from build123d import *

# Parameters (mm, degrees)
BOSS_EXTRUDE1_DEPTH             = 4
SKETCH2_W                       = 7.077783737
SKETCH2_H                       = 4
CUT_EXTRUDE1_DEPTH              = 2.402922374
BOSS_EXTRUDE2_START             = 4
BOSS_EXTRUDE2_DEPTH             = 4
SKETCH4_W                       = 7.077783737
SKETCH4_H                       = 8
CUT_EXTRUDE2_DEPTH              = 14.891763442
BOSS_EXTRUDE3_DEPTH             = 4
CUT_EXTRUDE3_DEPTH              = 6
SCALE1_SCALE                    = 0.6
SCALE2_SCALE                    = 1.1
CHAMFER2_ANGLE                  = 32.170804
CHAMFER3_ANGLE                  = 32.170804
CHAMFER4_ANGLE                  = 37.089833
SKETCH9_W                       = 9.052660039
SKETCH9_H                       = 40.26
BOSS_EXTRUDE4_DEPTH             = 10
BOSS_EXTRUDE4_DIRECTION_2_REACH = 42.714
FILLET1_R                       = 10


with BuildPart() as part:
    # Sketch1 → Boss-Extrude1 (new body)
    with BuildSketch(Plane(origin=(0, 2, 0), x_dir=(1, 0, 0), z_dir=(0, 1, 0))):
        with BuildLine():
            Line((17.294685816, -3.533576913), (17.294685816, 3.544206824))
            ThreePointArc((17.294685816, 3.544206824), (18.863114644, 8.869467938), (21.707787317, 13.636669664))
            ThreePointArc((21.707787317, 13.636669664), (21.87503123, 14.549681712), (21.219564158, 15.2068913))
            Line((21.219564158, 15.2068913), (10.486342132, 18.5754084))
            ThreePointArc((10.486342132, 18.5754084), (8.419274676, 21.892156447), (11.384661403, 24.437754026))
            Line((11.384661403, 24.437754026), (37.31661015, 24.437754026))
            Line((37.31661015, 24.437754026), (37.327723934, 22.056391914))
            ThreePointArc((37.327723934, 22.056391914), (43.539057979, 21.687528752), (49.402053126, 19.603777671))
            ThreePointArc((49.402053126, 19.603777671), (51.365484655, 19.664217825), (52.33016375, 21.37539012))
            Line((52.33016375, 21.37539012), (52.33016375, 27.503190326))
            ThreePointArc((52.33016375, 27.503190326), (45.90109867, 29.745314945), (39.134829344, 30.505314955))
            Line((39.134829344, 30.505314955), (-34.24156443, 30.505314955))
            Line((-34.24156443, 30.505314955), (-34.24156443, -30.494685045))
            Line((-34.24156443, -30.494685045), (39.134829344, -30.494685045))
            ThreePointArc((39.134829344, -30.494685045), (45.90109867, -29.734685035), (52.33016375, -27.492560416))
            Line((52.33016375, -27.492560416), (52.33016375, -21.36476021))
            ThreePointArc((52.33016375, -21.36476021), (51.365484655, -19.653587914), (49.402053126, -19.593147761))
            ThreePointArc((49.402053126, -19.593147761), (43.533593788, -21.678008046), (37.31661015, -22.044848399))
            Line((37.31661015, -22.044848399), (37.31661015, -24.427124116))
            Line((37.31661015, -24.427124116), (11.384661403, -24.427124116))
            ThreePointArc((11.384661403, -24.427124116), (8.419274676, -21.881526536), (10.486342132, -18.564778489))
            Line((10.486342132, -18.564778489), (21.219564158, -15.19626139))
            ThreePointArc((21.219564158, -15.19626139), (21.87503123, -14.539051801), (21.707787317, -13.626039753))
            ThreePointArc((21.707787317, -13.626039753), (18.863114644, -8.858838027), (17.294685816, -3.533576913))
        make_face()
    extrude(amount=-BOSS_EXTRUDE1_DEPTH)

    # Sketch2 → Cut-Extrude1 (cut)
    with BuildSketch(Plane(origin=(17.294685816, 0, 0), x_dir=(0, 0, -1), z_dir=(1, 0, 0))):
        with Locations((0.005314956, 0)):
            Rectangle(SKETCH2_W, SKETCH2_H)
    extrude(amount=-CUT_EXTRUDE1_DEPTH, mode=Mode.SUBTRACT)

    # Sketch3 → Boss-Extrude2 (add)
    with BuildSketch(Plane(origin=(0, 2, 0), x_dir=(-1, 0, 0), z_dir=(0, 1, 0)).offset(BOSS_EXTRUDE2_START)):
        with BuildLine():
            Line((-14.891763442, -3.544206824), (-14.891763442, 3.533576913))
            ThreePointArc((-14.891763442, 3.533576913), (-16.721112086, 9.887878597), (-20.183130277, 15.52153606))
            Line((-20.183130277, 15.52153606), (-10.486342132, 18.564778489))
            ThreePointArc((-10.486342132, 18.564778489), (-8.419274676, 21.881526536), (-11.384661403, 24.427124116))
            Line((-11.384661403, 24.427124116), (-37.31661015, 24.427124116))
            ThreePointArc((-37.31661015, 24.427124116), (-45.066931496, 23.76567922), (-52.219299017, 20.708126414))
            ThreePointArc((-52.219299017, 20.708126414), (-52.302252812, 21.031796649), (-52.33016375, 21.36476021))
            Line((-52.33016375, 21.36476021), (-52.33016375, 27.492560416))
            ThreePointArc((-52.33016375, 27.492560416), (-45.90109867, 29.734685035), (-39.134829344, 30.494685045))
            Line((-39.134829344, 30.494685045), (34.241565294, 30.494685045))
            Line((34.241565294, 30.494685045), (34.241565294, -30.505314955))
            Line((34.241565294, -30.505314955), (-39.134829344, -30.505314955))
            ThreePointArc((-39.134829344, -30.505314955), (-45.90109867, -29.745314945), (-52.33016375, -27.503190326))
            Line((-52.33016375, -27.503190326), (-52.33016375, -21.37539012))
            ThreePointArc((-52.33016375, -21.37539012), (-52.302252812, -21.04242656), (-52.219299017, -20.718756325))
            ThreePointArc((-52.219299017, -20.718756325), (-45.066931496, -23.77630913), (-37.31661015, -24.437754026))
            Line((-37.31661015, -24.437754026), (-11.384661403, -24.437754026))
            ThreePointArc((-11.384661403, -24.437754026), (-8.419274676, -21.892156447), (-10.486342132, -18.5754084))
            Line((-10.486342132, -18.5754084), (-20.183130277, -15.53216597))
            ThreePointArc((-20.183130277, -15.53216597), (-16.721112086, -9.898508508), (-14.891763442, -3.544206824))
        make_face()
    extrude(amount=-BOSS_EXTRUDE2_DEPTH)

    # Sketch4 → Cut-Extrude2 (cut)
    with BuildSketch(Plane(origin=(14.891763442, 0, 0), x_dir=(0, 0, -1), z_dir=(1, 0, 0))):
        with Locations((0.005314956, 2)):
            Rectangle(SKETCH4_W, SKETCH4_H)
    extrude(amount=-CUT_EXTRUDE2_DEPTH, mode=Mode.SUBTRACT)

    # Sketch5 → Boss-Extrude3 (add)
    with BuildSketch(Plane.XZ.offset(2)):
        with BuildLine():
            Line((37.31661015, 24.427124116), (11.384661403, 24.427124116))
            ThreePointArc((11.384661403, 24.427124116), (8.419274676, 21.881526536), (10.486342132, 18.564778489))
            Line((10.486342132, 18.564778489), (20.183130277, 15.52153606))
            ThreePointArc((20.183130277, 15.52153606), (16.721112086, 9.887878597), (14.891763442, 3.533576913))
            Line((14.891763442, 3.533576913), (0, 3.533576913))
            Line((0, 3.533576913), (0, -3.544206824))
            Line((0, -3.544206824), (14.891763442, -3.544206824))
            ThreePointArc((14.891763442, -3.544206824), (16.721112086, -9.898508508), (20.183130277, -15.53216597))
            Line((20.183130277, -15.53216597), (10.486342132, -18.5754084))
            ThreePointArc((10.486342132, -18.5754084), (8.419274676, -21.892156447), (11.384661403, -24.437754026))
            Line((11.384661403, -24.437754026), (37.31661015, -24.437754026))
            ThreePointArc((37.31661015, -24.437754026), (45.066931496, -23.77630913), (52.219299017, -20.718756325))
            ThreePointArc((52.219299017, -20.718756325), (52.302252812, -21.04242656), (52.33016375, -21.37539012))
            Line((52.33016375, -21.37539012), (52.33016375, -27.503190326))
            ThreePointArc((52.33016375, -27.503190326), (45.90109867, -29.745314945), (39.134829344, -30.505314955))
            Line((39.134829344, -30.505314955), (-34.241565294, -30.505314955))
            Line((-34.241565294, -30.505314955), (-34.241565294, 30.494685045))
            Line((-34.241565294, 30.494685045), (39.134829344, 30.494685045))
            ThreePointArc((39.134829344, 30.494685045), (45.90109867, 29.734685035), (52.33016375, 27.492560416))
            Line((52.33016375, 27.492560416), (52.33016375, 21.36476021))
            ThreePointArc((52.33016375, 21.36476021), (52.302252812, 21.031796649), (52.219299017, 20.708126414))
            ThreePointArc((52.219299017, 20.708126414), (45.066931496, 23.76567922), (37.31661015, 24.427124116))
        make_face()
    extrude(amount=BOSS_EXTRUDE3_DEPTH)

    # Sketch6 → Cut-Extrude3 (cut)
    with BuildSketch(Plane(origin=(0, 6, 0), x_dir=(-1, 0, 0), z_dir=(0, 1, 0))):
        with BuildLine():
            Line((34.241565294, 21.494683919), (0.615148415, 21.494683919))
            ThreePointArc((0.615148415, 21.494683919), (-0.40252933, 16.590516303), (-3.333426268, 12.528943807))
            ThreePointArc((-3.333426268, 12.528943807), (0.609678883, 11.977798965), (4.155422589, 10.166848817))
            ThreePointArc((4.155422589, 10.166848817), (5.046731763, 9.106387113), (5.366566942, 7.758530841))
            Line((5.366566942, 7.758530841), (5.366566942, -7.769160752))
            ThreePointArc((5.366566942, -7.769160752), (5.046731763, -9.117017023), (4.155422589, -10.177478728))
            ThreePointArc((4.155422589, -10.177478728), (0.609678883, -11.988428875), (-3.333426268, -12.539573718))
            ThreePointArc((-3.333426268, -12.539573718), (-0.402529103, -16.601146729), (0.615148409, -21.505314955))
            Line((0.615148409, -21.505314955), (34.241565294, -21.505314955))
            Line((34.241565294, -21.505314955), (34.241565294, 21.494683919))
        make_face()
    extrude(amount=-CUT_EXTRUDE3_DEPTH, mode=Mode.SUBTRACT)


with BuildPart() as part_1:
    # Scale1: scaled about (-0.143748337, -0.76143553, -0.005277361)
    add(part.part.scale(SCALE1_SCALE).moved(Location((-0.057499335, -0.304574212, -0.002110944))))


with BuildPart() as part_2:
    # Scale2: scaled about (-0.143748337, -0.76143553, -0.005277361)
    add(part_1.part.scale(SCALE2_SCALE).moved(Location((0.014374834, 0.076143553, 0.000527736))))

    # Chamfer2: read off the stored shape, not the designer's step
    # Chamfer2 outline → Chamfer2 (revolve, cut)
    with BuildSketch(Plane(origin=(25.780112964, 0, -0.005302173), x_dir=(-0.9894243177123465, 0, 0.14505005866754295), z_dir=(-0.14505005866754295, 0, -0.9894243177123465))):
        Polygon((16.1025, -1.578888079), (14.602499776, -0.078887855), (14.602499776, -1.578888079), align=None)
    revolve(axis=Axis((25.780112964, 0, -0.005302173), (0, 1, 0)), revolution_arc=CHAMFER2_ANGLE, mode=Mode.SUBTRACT)

    # Chamfer3: read off the stored shape, not the designer's step
    # Chamfer3 outline → Chamfer3 (revolve, cut)
    with BuildSketch(Plane(origin=(25.780112964, 0, -0.005302173), x_dir=(-0.7602814738740017, 0, -0.6495937811309278), z_dir=(0.6495937811309278, 0, -0.7602814738740017))):
        Polygon((16.1025, -1.578888079), (14.602499776, -0.078887855), (14.602499776, -1.578888079), align=None)
    revolve(axis=Axis((25.780112964, 0, -0.005302173), (0, 1, 0)), revolution_arc=CHAMFER3_ANGLE, mode=Mode.SUBTRACT)

    # Chamfer4: read off the stored shape, not the designer's step
    # Chamfer4 outline → Chamfer4 (revolve, cut)
    with BuildSketch(Plane(origin=(25.780112964, 0, -0.005302173), x_dir=(0.5358984482336857, 0, -0.8442824486987324), z_dir=(0.8442824486987324, 0, 0.5358984482336857))):
        Polygon((16.1025, -1.578888079), (14.602495102, -0.078883181), (14.602495102, -1.578888079), align=None)
    revolve(axis=Axis((25.780112964, 0, -0.005302173), (0, 1, 0)), revolution_arc=CHAMFER4_ANGLE, mode=Mode.SUBTRACT)

    # Chamfer5: read off the stored shape, not the designer's step
    # Chamfer5 outline → Chamfer5 (revolve, cut)
    with BuildSketch(Plane(origin=(25.780112964, 0, -0.005302173), x_dir=(1, 0, 0), z_dir=(0, 0, 1))):
        Polygon((16.1025, -1.578888079), (14.602495102, -0.078883181), (14.602495102, -1.578888079), align=None)
    revolve(axis=Axis((25.780112964, 0, -0.005302173), (0, 1, 0)), mode=Mode.SUBTRACT)

    # Sketch9 → Boss-Extrude4 (add)
    with BuildSketch(Plane(origin=(0, 3.701111921, 0), x_dir=(1, 0, 0), z_dir=(0, 1, 0))):
        with Locations((-18.121977477, 0.005302173)):
            Rectangle(SKETCH9_W, SKETCH9_H)
    extrude(amount=BOSS_EXTRUDE4_DEPTH)

    # Boss-Extrude4 direction 2: up to this face of the body (flat: up to its plane)
    boss_extrude4_direction_2_end = Plane(part_2.part.faces().sort_by_distance((-12.071218374, -0.25888808, -0.005302566))[0])
    # Sketch9 → Boss-Extrude4 direction 2 (add, up to the picked face)
    with BuildSketch(Plane(origin=(0, 3.701111921, 0), x_dir=(1, 0, 0), z_dir=(0, 1, 0)), mode=Mode.PRIVATE) as boss_extrude4_direction_2_sk1:
        with Locations((-18.121977477, 0.005302173)):
            Rectangle(SKETCH9_W, SKETCH9_H)
    boss_extrude4_direction_2_tool1 = split(extrude(boss_extrude4_direction_2_sk1.sketch, amount=-BOSS_EXTRUDE4_DIRECTION_2_REACH, mode=Mode.PRIVATE), bisect_by=boss_extrude4_direction_2_end, keep=Keep.BOTH, mode=Mode.PRIVATE)
    add(boss_extrude4_direction_2_tool1.solids().sort_by(Axis((-18.121977, 3.701112, -0.005302), (0, -1, 0)))[0])

    # Fillet1
    fillet1_edges = [part_2.edges().sort_by_distance(p)[0] for p in [
        (-13.595647458, 3.701111921, -17.165302173),
    ]]
    fillet(fillet1_edges, radius=FILLET1_R - 0.0001)  # a hair under: the kernel refuses the full size


solid = part_2.part
Geometry: final body of the model. Coordinates: model frame, mm. A direction names the side the tool comes from. Give positions to 0.01 mm unless a question says otherwise; leave off trailing zeros. Write each loop counter-clockwise with the first axis right and the second up, starting at its lowest first coordinate (ties: lowest second). Pieces come first, ordered by that corner, then holes. Notation, with made-up numbers: M 70,-38 L 100,-38 A23 ccw 100,-20 Z; hole C 2,-38.5 d1. An arc over 180 degrees is marked long. Answer in a Markdown table with one row per item. Add a question column.
(1) Section B-B on z = 17.5. Return loops of the section in (x, y), and give its area (3 significant figures).
(2) Section C-C on x = 9. Return loops of the section in (y, z).
(3) Ray query, line 1 (Z direction, x = 23, y = 2.25); line 2 (Z direction, x = 7, y = -1.75); line 3 (Z direction, x = -12, y = 3.5). Return the intervals inside material, ascending.
(4) Section D-D on y = 11.75. Return loops of the section in (x, z).
(5) Mould query, pull axis X, two halves, no side actions, for faces 1 (the flat face through (12, 1.061, -6)), 2 (the conical face through (11.99, -0.65, -6.33)), 3 (the flat face through (16, 0, 16.12)). Classes: +X half, -X half, draft (parallel to the pull), parting line (faces both ways), or undercut.
(6) First-contact query: pin 1 (1 mm diameter, centred on x = 30, z = -14, fed in from +Y); pin 2 (10 mm diameter, centred on y = -1, z = 1, fed in from +X); pin 3 (5 mm diameter, centred on x = 13, z = 6, fed in from +Y). Flat tips, straight axial feed; report the tip coordinate or a pass-through.
(7) Section A-A on x = 18. Return loops of the section in (y, z).
(8) Reachability of faces 4 (the cylindrical face through (29.765, 2.4, -15.677)), 5 (the cylindrical face through (5.5, -0.2, -14.4)), 6 (the cylindrical face through (10.962, 2.4, 6.468)) from +Z, -Z, +X, -X, +Y, -Y: full face, straight path, thin tool, end or side. Return the list, or none.
Result set:
| question | item | result |
|---|---|---|
| 1 | outline | M -22.65,-4.22 L 34.49,-4.22 L 34.49,3.7 L -13.6,3.7 L -13.6,13.7 L -22.65,13.7 Z |
| 1 | area | 543 mm^2 |
| 2 | outline | M -4.22,-20.14 L 3.7,-20.14 L 3.7,-16.13 L -4.22,-16.13 Z; M -4.22,-11.59 L 3.7,-11.59 L 3.7,-2.34 L -4.22,-2.34 Z; M -4.22,2.33 L 3.7,2.33 L 3.7,11.58 L -4.22,11.58 Z; M -4.22,16.12 L 3.7,16.12 L 3.7,20.12 L -4.22,20.12 Z |
| 3 | line 1 | z = -20.14 to -16.13, 16.12 to 20.12 |
| 3 | line 2 | z = -20.14 to -16.08, -12.22 to -2.34, 2.33 to 12.21, 16.06 to 20.12 |
| 3 | line 3 | z = -20.14 to -14.2, 14.18 to 20.12 |
| 4 | outline | M -22.65,-20.14 L -13.4,-20.14 L -13.4,-14.2 L -13.6,-14.2 L -13.6,20.12 L -22.65,20.12 Z |
| 5 | face 1 | draft |
| 5 | face 2 | +X half |
| 5 | face 3 | undercut |
| 6 | pin 1 | stops at y = 1.06 |
| 6 | pin 2 | stops at x = 12.43 |
| 6 | pin 3 | stops at y = 3.7 |
| 7 | outline | M -4.22,-20.14 L 3.7,-20.14 L 3.7,-16.13 L -4.22,-16.13 Z; M -4.22,16.12 L 3.7,16.12 L 3.7,20.12 L -4.22,20.12 Z |
| 8 | face 4 | +Y |
| 8 | face 5 | +Y, -Y |
| 8 | face 6 | +X, +Y |
